```python
from build123d import *

# Parameters (mm, degrees)
F0_W      = 60
F0_H      = 40
F1_DEPTH  = 50
F2_W      = 20
F2_H      = 10
F3_DEPTH  = 60
F7_DEPTH  = 10
F10_DEPTH = 25
F11_R     = 35
F12_DEPTH = 10
F15_DEPTH = 50
F17_DEPTH = 50.001
F19_DEPTH = 20.1260024637


with BuildPart() as f1:
    # F0 (on Top) → F1 (new body)
    with BuildSketch(Plane.XY):
        with Locations((30, 20)):
            Rectangle(F0_W, F0_H)
    extrude(amount=F1_DEPTH)

    # F2 (on face) → F3 (cut, through all)
    with BuildSketch(Plane.YZ.offset(60)):
        with Locations((20, 5)):
            Rectangle(F2_W, F2_H)
    extrude(amount=-F3_DEPTH, mode=Mode.SUBTRACT)

    # F6 (on face) → F7 (cut, through all)
    with BuildSketch(Plane(origin=(0, 0, 0), x_dir=(0, -1, 0), z_dir=(-1, 0, 0))):
        Polygon((0, 40), (0, 50), (-20, 50), align=None)
    extrude(amount=-F7_DEPTH, mode=Mode.SUBTRACT)

    # F9 (on offset) → F10 (cut, through all)
    with BuildSketch(Plane.YZ.offset(20)):
        Polygon((20, 50), (0, 50), (0, 30), align=None)
    extrude(amount=F10_DEPTH, mode=Mode.SUBTRACT)

    # F11 (on offset) → F12 (cut, through all)
    with BuildSketch(Plane.YZ.offset(10)):
        with Locations((0, 50)):
            Circle(F11_R)
    extrude(amount=F12_DEPTH, mode=Mode.SUBTRACT)

    # F14 (on offset) → F15 (cut)
    with BuildSketch(Plane.XY.offset(50)):
        Polygon((30.0937518477, 0), (45.0937518477, 0), (45.0937518477, 20), align=None)
    extrude(amount=-F15_DEPTH, mode=Mode.SUBTRACT)

    # F16 (on face) → F17 (cut, through all)
    with BuildSketch(Plane.XY.offset(50)):
        Polygon((60, 0), (60, 30), (45.0937518477, 20), (45.0937518477, 0), align=None)
    extrude(amount=-F17_DEPTH, mode=Mode.SUBTRACT)

    # F18 (on face) → F19 (cut, through all)
    with BuildSketch(Plane(origin=(0, 40, 0), x_dir=(-1, 0, 0), z_dir=(0, 1, 0))):
        Polygon((-45, 50), (-60, 50), (-60, 10), align=None)
    extrude(amount=-F19_DEPTH, mode=Mode.SUBTRACT)


solid = f1.part
```
Design review of the part built by this model. Coordinates are the model's own, in mm. A direction names the side the tool comes from. Coordinates: 2 decimals unless noted, no trailing zeros. Write each loop counter-clockwise with the first axis right and the second up, starting at its lowest first coordinate (ties: lowest second). Pieces come first, ordered by that corner, then holes.
1) Add section C-C (y = 14). Write out the cut boundary in (x, z), plus the area to 3 significant figures.
2) Insertion check: pin 1 (1.5 mm diameter, centred on y = 22.5, z = 40, fed in from +X); pin 2 (1.5 mm diameter, centred on y = 17, z = 27, fed in from -X); pin 3 (8 mm diameter, centred on x = 28, y = 21.5, fed in from -Z). Each pin has a flat end and moves straight along its axis. Give the tip position at first contact, or say it passes through.
3) Add section D-D (x = 23.5). Write out the cut boundary in (y, z).
4) Add section A-A (x = 17.5). Write out the cut boundary in (y, z).
5) Machinability: for faces 1 (the flat face through (19, 10, 5)), 2 (the flat face through (20, 17, 33)), 3 (the flat face through (22, 30, 50)), which of the approach directions +Z, -Z, +X, -X, +Y, -Y give a long, thin tool a straight path to every point of the face, cutting with its end or side? Answer none if there is none.
6) To check wall thickness, follow L1, parallel to Y at x = 25.5, z = 3.5; L2, parallel to X at y = 12, z = 21; L3, parallel to X at y = 27.5, z = 36. State the ranges of each line that lie inside material, in increasing order.
7) Add section B-B (z = 22.5). Write out the cut boundary in (x, y), plus the area to 3 significant figures.
8) Mouldability with a two-part tool opening along X and no side actions: class faces 4 (the flat face through (24, 20, 10)), 5 (the flat face through (10, 17, 33)), 6 (the flat face through (52.605, 32.314, 29.72)) as +X half, -X half, draft (parallel to the pull), parting line (faces both ways), or undercut.
Check result:
1. outline: (0, 10) - (40.59, 10) - (40.59, 44) - (20, 44) - (20, 17.92) - (10, 17.92) - (10, 47) - (0, 47) - close
1. area: 1,150 mm2
2. pin 1: stops at x = 49.03
2. pin 2: stops at x = 0
2. pin 3: stops at z = 10
3. outline: (0, 0) - (10, 0) - (10, 10) - (30, 10) - (30, 0) - (40, 0) - (40, 50) - (20, 50) - (0, 30) - close
4. outline: (0, 0) - (10, 0) - (10, 10) - (30, 10) - (30, 0) - (40, 0) - (40, 50) - (35, 50) arc R35 cw to (0, 15) - close
5. face 1: -Z, +X, -X
5. face 2: +Z, -Y
5. face 3: +Z, +X, -X, +Y, -Y
6. L1: y = 0 to 10, 30 to 40
6. L2: x = 0 to 10, 20 to 39.09
6. L3: x = 0 to 10, 20 to 50.25
7. outline: (0, 0) - (10, 0) - (10, 21.65) - (20, 21.65) - (20, 0) - (30.09, 0) - (45.09, 20) - (55.31, 26.86) - (55.31, 40) - (0, 40) - close
7. area: 1,610 mm2
8. face 4: draft
8. face 5: undercut
8. face 6: +X half
